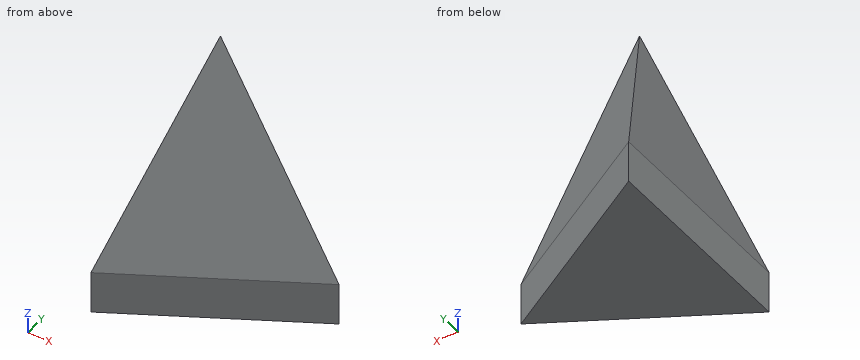
```python
from build123d import *

# Parameters (mm, degrees)
F1_DEPTH = 25


with BuildPart() as f1:
    # F0 (on Top) → F1 (new body)
    with BuildSketch(Plane.XY):
        Polygon((70.286689, -1.822083), (-33.565374, 61.7811), (-36.721315, -59.959017), align=None)
    extrude(amount=F1_DEPTH)

    # F1_face (on face) → F4 section 0
    with BuildSketch(Plane.XY.offset(25), mode=Mode.PRIVATE) as f4_s0:
        Polygon((-36.721315, -59.959017), (70.286689, -1.822083), (-33.565374, 61.7811), align=None)
    loft([f4_s0.sketch, Vertex(0, 0, 150)])


solid = f1.part
```
Work out the finished part from the listing and answer in its coordinate system (mm). Give positions to 0.01 mm unless a question says otherwise; leave off trailing zeros. Order: outer loops, then holes, each group sorted by start corner. A loop starts at its lowest first (then second) coordinate and runs counter-clockwise, first axis right, second up. Notation, with made-up numbers: (77.25, 77.25) -> (119.25, 77.25) arc R25 ccw to (119.25, 103.25) -> close; hole circle Ø11 at (66, 81.25). An arc over 180 degrees is marked (long way). Answer as CSV lines item,"result". Start each with the question number.
(1) Section A-A, the plane y = -40 is taken. Write down the section's boundary in (x, z), plus the area to 3 significant figures.
(2) Section B-B, the plane x = 39 is taken. Write down the section's boundary in (y, z), plus the area to 3 significant figures.
(3) Section D-D, the plane z = 110 is taken. Write down the section's boundary in (x, y).
(4) Consider line 1 along X through (y, z) = (-25.5, 18.5); line 2 along Y through (x, z) = (60, 28.5); line 3 along Y through (x, z) = (-10, 108). Determine where each line is inside the solid, lowest interval first.
(5) Each of these flat-tipped pins is pushed along its axis until it touches: pin 1 Ø8 at (x, y) = (18, 39.5) entering from +Z; pin 2 Ø6 at (y, z) = (-36.5, 74) entering from +X; pin 3 Ø12 at (x, z) = (-4, 81.5) entering from -Y; pin 4 Ø2 at (y, z) = (16, 30.5) entering from +X. Where does it stop, or does it pass through?
(6) Section C-C, the plane z = 30.5 is taken. Write down the section's boundary in (x, y), plus the area to 3 significant figures.
Entries:
1,outline,"(-36.2, 0) -> (0.02, 0) -> (0.02, 25) -> (-24.5, 66.61) -> (-36.2, 25) -> close"
1,area,"1,660 mm²"
2,outline,"(-18.82, 0) -> (17.34, 0) -> (17.34, 25) -> (-1.01, 80.64) -> (-18.82, 25) -> close"
2,area,"1,910 mm²"
3,outline,"(-11.75, -19.19) -> (22.49, -0.58) -> (-10.74, 19.77) -> close"
4,line 1,"-35.83 to 26.7"
4,line 2,"-6.29 to 3.32"
4,line 3,"-18.88 to 19.98"
5,pin 1,"through"
5,pin 2,"x = -16.61"
5,pin 3,"y = -27.88"
5,pin 4,"x = 39.94"
6,outline,"(-35.11, -57.32) -> (67.19, -1.74) -> (-32.09, 59.06) -> close"
6,area,"5,870 mm²"
